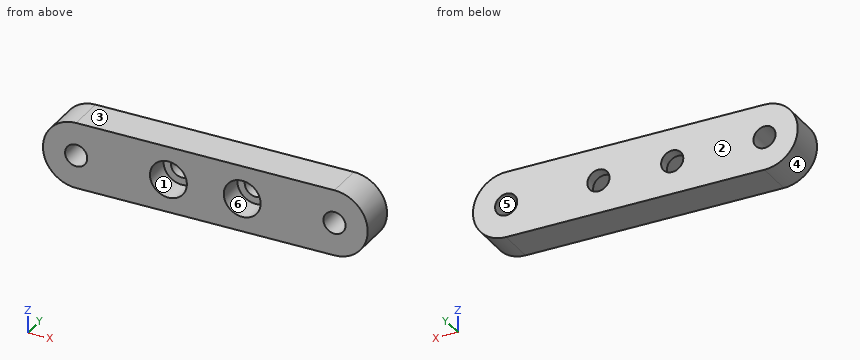
from build123d import *

# Parameters (mm, degrees)
SKETCH2_R           = 3
BOSS_EXTRUDE1_DEPTH = 10
SKETCH3_R           = 5
CUT_EXTRUDE1_DEPTH  = 7


with BuildPart() as part:
    # Sketch2 → Boss-Extrude1 (new body)
    with BuildSketch(Plane(origin=(0, 0, 0), x_dir=(1, 0, 0), z_dir=(0, 1, 0))):
        with BuildLine():
            ThreePointArc((25, -9), (34, 0), (25, 9))
            Line((25, 9), (-45, 9))
            ThreePointArc((-45, 9), (-54, 0), (-45, -9))
            Line((-45, -9), (25, -9))
        make_face()
        with Locations((-20, 0)):
            Circle(SKETCH2_R, mode=Mode.SUBTRACT)
        Circle(SKETCH2_R, mode=Mode.SUBTRACT)
        with Locations((25, 0)):
            Circle(SKETCH2_R, mode=Mode.SUBTRACT)
        with Locations((-45, 0)):
            Circle(SKETCH2_R, mode=Mode.SUBTRACT)
    extrude(amount=BOSS_EXTRUDE1_DEPTH)

    # Sketch3 → Cut-Extrude1 (cut)
    with BuildSketch(Plane.XZ):
        with Locations((-20, 0)):
            Circle(SKETCH3_R)
        Circle(SKETCH3_R)
    extrude(amount=-CUT_EXTRUDE1_DEPTH, mode=Mode.SUBTRACT)


solid = part.part
CAD build for the part. Positions are in the model's coordinates, mm. Face numbers are marked on the shaded views. A direction names the side the tool comes from. Round coordinates to 2 decimals unless told otherwise and drop trailing zeros. Write each loop counter-clockwise with the first axis right and the second up, starting at its lowest first coordinate (ties: lowest second). Pieces come first, ordered by that corner, then holes. Notation, with made-up numbers: M 76,83 L 93,83 A17 ccw 93,103 Z; hole C 64,45 d10. An arc over 180 degrees is marked long. Put each result on its own line as item: value. Start each with the question number.
1) Saw through at C-C, the plane x = 0. Write the cut outline in (y, z).
2) Drill centre lines: probe 1 along X at (y, z) = (8.25, 0); probe 2 along X at (y, z) = (2.5, 2.5); probe 3 along Z at (x, y) = (0, 2.75). Where is each one in solid material? Low to high. Write a range as [from, to].
3) Pin check, flat tips, straight feed: pin 1 Ø1.5 at (y, z) = (4.5, 6.5) entering from +X; pin 2 Ø3 at (y, z) = (5, -2.5) entering from -X; pin 3 Ø2 at (y, z) = (3, -7) entering from +X; pin 4 Ø1.5 at (y, z) = (3.5, -0.5) entering from -X. Stop position of each tip, or through.
4) 3-axis set-ups, long thin cutter, end or side, ignore diameter. For the marked faces 1 and 2: which of +Z, -Z, +X, -X, +Y, -Y reach the whole face in a straight line?
5) Saw through at A-A, the plane z = 0. Write the cut outline in (x, y), and give its area (3 significant figures).
6) Pull direction X, two halves, no side cores. Call the marked faces 3, 4, 5 and 6: pulls with the +X half, pulls with the -X half, needs draft (parallel to the pull), parting line crosses it, or undercut.
7) Saw through at B-B, the plane y = 2.25. Write the cut outline in (x, z).
8) Saw through at D-D, the plane x = -16. Write the cut outline in (y, z).
Resolved:
1. outline: M 0,-9 L 10,-9 L 10,-3 L 7,-3 L 7,-5 L 0,-5 Z; M 0,5 L 7,5 L 7,3 L 10,3 L 10,9 L 0,9 Z
2. probe 1: [-54, -48], [-42, -23], [-17, -3], [3, 22], [28, 34]
2. probe 2: [-53.65, -46.66], [-43.34, -24.33], [-15.67, -4.33], [4.33, 23.34], [26.66, 33.65]
2. probe 3: [-9, -5], [5, 9]
3. pin 1: x = 31.92
3. pin 2: x = -53.94
3. pin 3: x = 31.71
3. pin 4: x = -54
4. face 1: -Y
4. face 2: +Z, -Z, +X, -X, +Y
5. outline: M -54,0 L -48,0 L -48,10 L -54,10 Z; M -42,0 L -25,0 L -25,7 L -23,7 L -23,10 L -42,10 Z; M -17,7 L -15,7 L -15,0 L -5,0 L -5,7 L -3,7 L -3,10 L -17,10 Z; M 3,7 L 5,7 L 5,0 L 22,0 L 22,10 L 3,10 Z; M 28,0 L 34,0 L 34,10 L 28,10 Z
5. area: 584 mm²
6. face 3: needs draft
6. face 4: pulls with the -X half
6. face 5: undercut
6. face 6: undercut
7. outline: M -45,-9 L 25,-9 A9 ccw 25,9 L -45,9 A9 ccw Z; hole C -45,0 d6; hole C -20,0 d10; hole C 0,0 d10; hole C 25,0 d6
8. outline: M 0,-9 L 10,-9 L 10,9 L 0,9 L 0,3 L 7,3 L 7,-3 L 0,-3 Z
